Read the model definition and answer for the solid it produces. Units are mm, in the model's axes. Face numbers are marked on the shaded views. A direction names the side the tool comes from. Coordinates: 2 decimals unless noted, no trailing zeros. Order: outer loops, then holes, each group sorted by start corner. A loop starts at its lowest first (then second) coordinate and runs counter-clockwise, first axis right, second up. Notation, with made-up numbers: M -20.75,73 L 31.25,73 A14 ccw 31.25,89 Z; hole C 5.25,-23.75 d3. An arc over 180 degrees is marked long. Put each result on its own line as item: value.
from build123d import *

# Parameters (mm, degrees)
F0_W        = 88.9
F0_H        = 165.1
F1_DEPTH    = 6.35
F2_DEPTH    = 25.4
F3_DEPTH    = 50.8
F4_SIZE2    = 7.3323484187
F4_SIZE     = 12.7
F5_C1_SIZE2 = 12.7
F5_C1_SIZE  = 7.3323484187
F5_C2_SIZE2 = 7.3323484187
F5_C2_SIZE  = 12.7
F5_C3_SIZE2 = 12.7
F5_C3_SIZE  = 7.3323484187
F5_C4_SIZE2 = 7.3323484187
F5_C4_SIZE  = 12.7


with BuildPart() as f1:
    # F0 (on Top) → F1 (new body)
    with BuildSketch(Plane.XY):
        Rectangle(F0_W, F0_H)
        Polygon((0, 76.2), (38.1, 76.2), (38.1, -38.1), (38.1, -76.2), (0, -76.2), (-38.1, -76.2), (-38.1, 38.1), (-38.1, 76.2), align=None, mode=Mode.SUBTRACT)
    extrude(amount=F1_DEPTH)

    # F0 (on Top) → F2 (join)
    with BuildSketch(Plane.XY):
        with BuildLine():
            Line((38.1, -38.1), (38.1, 76.2))
            Line((38.1, 76.2), (0, 76.2))
            Line((0, 76.2), (0, 50.8))
            ThreePointArc((0, 50.8), (-3.7197438789, 41.8197438789), (-12.7, 38.1))
            Line((-12.7, 38.1), (-38.1, 38.1))
            Line((-38.1, 38.1), (-38.1, -76.2))
            Line((-38.1, -76.2), (0, -76.2))
            Line((0, -76.2), (0, -50.8))
            ThreePointArc((0, -50.8), (3.7197438789, -41.8197438789), (12.7, -38.1))
            Line((12.7, -38.1), (38.1, -38.1))
        make_face()
    extrude(amount=F2_DEPTH)

    # F0 (on Top) → F3 (join)
    with BuildSketch(Plane.XY):
        with BuildLine():
            Line((0, 50.8), (0, 76.2))
            Line((0, 76.2), (-38.1, 76.2))
            Line((-38.1, 76.2), (-38.1, 38.1))
            Line((-38.1, 38.1), (-12.7, 38.1))
            ThreePointArc((-12.7, 38.1), (-3.7197438789, 41.8197438789), (0, 50.8))
        make_face()
        with BuildLine():
            Line((38.1, -76.2), (38.1, -38.1))
            Line((38.1, -38.1), (12.7, -38.1))
            ThreePointArc((12.7, -38.1), (3.7197438789, -41.8197438789), (0, -50.8))
            Line((0, -50.8), (0, -76.2))
            Line((0, -76.2), (38.1, -76.2))
        make_face()
    extrude(amount=F3_DEPTH)

    # F4
    f4_edges = [f1.edges().sort_by_distance(p)[0] for p in [
        (-38.1, -19.05, 25.4),
        (19.05, 76.2, 25.4),
        (38.1, 19.05, 25.4),
        (-19.05, -76.2, 25.4),
    ]]
    f4_side = f1.faces().sort_by_distance((0, 0, 25.4))[0]
    chamfer(f4_edges, length=F4_SIZE, length2=F4_SIZE2, reference=f4_side)

    # F5: chamfer of 12.7 x 7.3323484187 on 4 edges, made by hand

    # F5_c1
    f5_c1_edges = [f1.edges().sort_by_distance(p)[0] for p in [
        (-38.1, 57.15, 50.8),
    ]]
    f5_c1_side = f1.faces().sort_by_distance((-38.1, 57.15, 50.6533530316))[0]
    chamfer(f5_c1_edges, length=F5_C1_SIZE, length2=F5_C1_SIZE2, reference=f5_c1_side)

    # F5_c2
    f5_c2_edges = [f1.edges().sort_by_distance(p)[0] for p in [
        (19.05, -76.2, 50.8),
    ]]
    f5_c2_side = f1.faces().sort_by_distance((19.05, -76.2, 50.6533530316))[0]
    chamfer(f5_c2_edges, length=F5_C2_SIZE, length2=F5_C2_SIZE2, reference=f5_c2_side)

    # F5_c3
    f5_c3_edges = [f1.edges().sort_by_distance(p)[0] for p in [
        (-12.7, 76.2, 50.8),
    ]]
    f5_c3_side = f1.faces().sort_by_distance((-12.7, 76.2, 50.6533530316))[0]
    chamfer(f5_c3_edges, length=F5_C3_SIZE, length2=F5_C3_SIZE2, reference=f5_c3_side)

    # F5_c4
    f5_c4_edges = [f1.edges().sort_by_distance(p)[0] for p in [
        (38.1, -53.4838257906, 50.8),
    ]]
    f5_c4_side = f1.faces().sort_by_distance((38.1, -53.4838257906, 50.6533530316))[0]
    chamfer(f5_c4_edges, length=F5_C4_SIZE, length2=F5_C4_SIZE2, reference=f5_c4_side)


solid = f1.part
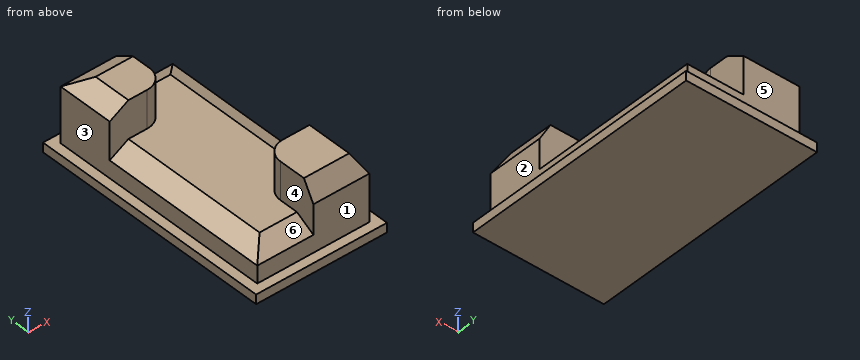
Q1. A tool of negligible diameter and unlimited length cuts with its end or side. For the marked faces 1, 2 and 3, from which of +Z, -Z, +X, -X, +Y, -Y can it reach the whole face along a straight path? Write none if from no direction.
Answers below:
face 1: +Z, +X, -X, -Y
face 2: +Z, +X, +Y, -Y
face 3: +Z, -X, +Y, -Y
Q2. Consider line 1 along Z through (x, y) = (-24.5, -25.5); line 2 along Y through (x, z) = (-12.5, 11); line 3 along Y through (x, z) = (20, 35). Determine where each line is inside the solid, lowest interval first.
Answers below:
line 1: z = 0 to 25.4
line 2: y = -76.2 to 76.2
line 3: y = -76.2 to -38.1
Q3. Find section A-A on z = 35. Write down the section's boundary in (x, y), plus the area to 3 significant figures.
Answers below:
outline: M -38.1,38.1 L -12.7,38.1 A12.7 ccw 0,50.8 L 0,76.2 L -38.1,76.2 Z; M 0,-76.2 L 38.1,-76.2 L 38.1,-38.1 L 12.7,-38.1 A12.7 ccw 0,-50.8 Z
area: 2,830 mm^2
Q4. Find section D-D on z = 23. Write down the section's boundary in (x, y), plus the area to 3 significant figures.
Answers below:
outline: M -38.1,38.1 L -29.56,38.1 L -29.56,-67.66 L 0,-67.66 L 0,-76.2 L 38.1,-76.2 L 38.1,-38.1 L 29.56,-38.1 L 29.56,67.66 L 0,67.66 L 0,76.2 L -38.1,76.2 Z
area: 9,150 mm^2
Q5. Given pin 1 (12.5 mm diameter, centred on x = -29, z = 31.5, fed in from -Y); pin 2 (2 mm diameter, centred on x = -16.5, y = -5.5, fed in from +Z); pin 3 (9.5 mm diameter, centred on x = -12.5, z = 22.5, fed in from -Y), each flat-ended and moving along its own axis, determine where each tip first touches the part or whether it passes through.
Answers below:
pin 1: stops at y = 38.1
pin 2: stops at z = 25.4
pin 3: stops at y = -76.2
Q6. For a pull along Y with two mould halves and no side action, classify the marked faces 4, 5 and 6 as +Y half, -Y half, draft (parallel to the pull), parting line (faces both ways), or undercut.
Answers below:
face 4: draft
face 5: +Y half
face 6: -Y half
Q7. Find section B-B on x = -15. Write down the section's boundary in (y, z).
Answers below:
outline: M -82.55,0 L 82.55,0 L 82.55,6.35 L 76.2,6.35 L 76.2,43.47 L 63.5,50.8 L 38.1,50.8 L 38.1,25.4 L -63.5,25.4 L -76.2,18.07 L -76.2,6.35 L -82.55,6.35 Z
Q8. Find section C-C on y = 22. Write down the section's boundary in (x, z).
Answers below:
outline: M -44.45,0 L 44.45,0 L 44.45,6.35 L 38.1,6.35 L 38.1,18.07 L 25.4,25.4 L -25.4,25.4 L -38.1,18.07 L -38.1,6.35 L -44.45,6.35 Z
